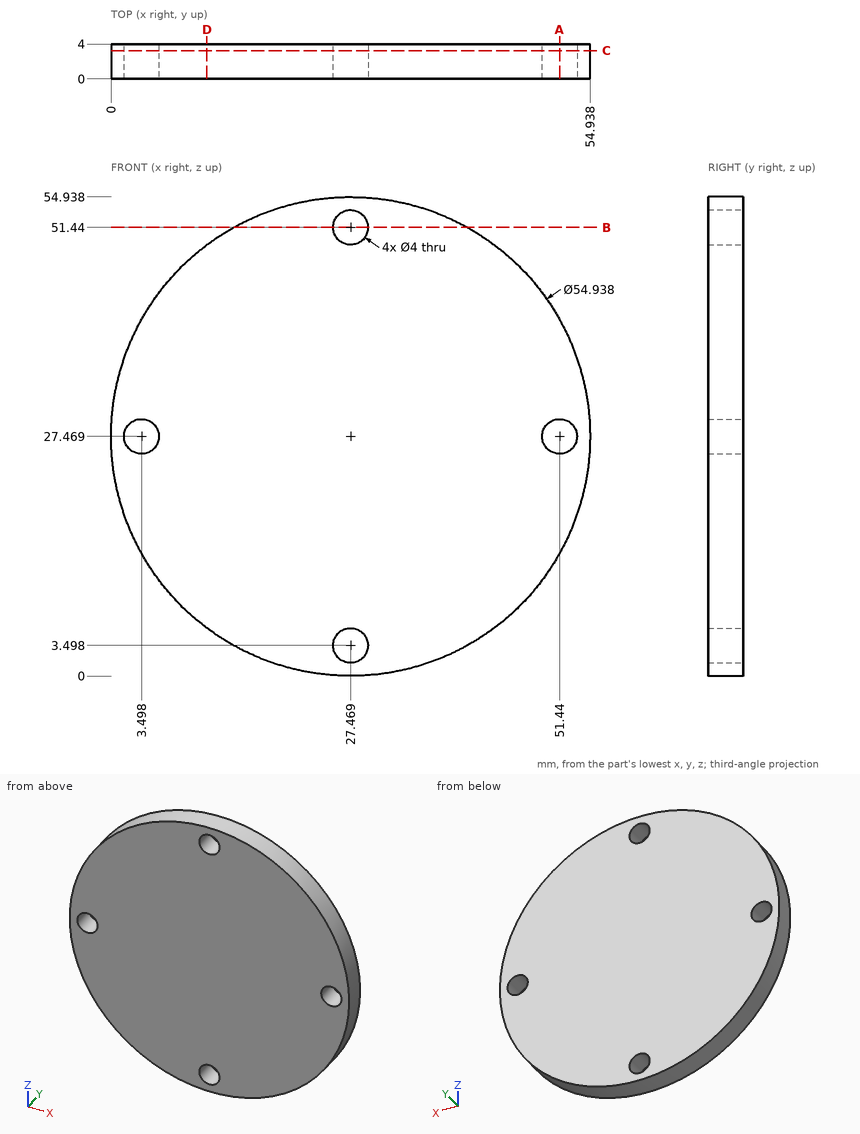
Can you work these out from the drawing? Everything is in mm from the part's minimum corner. Round coordinates to 2 decimals unless told otherwise and drop trailing zeros. Loops run counter-clockwise (first coordinate to the right, second up) from the corner with the lowest first, then second, coordinate; pieces in that order, holes last. Notation, with made-up numbers: (-3, 22) -> (8, 22) arc R23 ccw to (8, 32) -> close; hole circle Ø9 at (-10, 15.5). An arc over 180 degrees is marked (long way). Use CSV: the item, a comma, the result in double quotes.
(1) Suppose I cut it at A-A on x = 51.44. Write out the boundary of the cut face in (y, z).
Return value:
outline,"(0, 14.05) -> (4, 14.05) -> (4, 25.47) -> (0, 25.47) -> close; (0, 29.47) -> (4, 29.47) -> (4, 40.88) -> (0, 40.88) -> close"
(2) Will these pins go through, and if not, where does the flat tip stop? pin 1 Ø2.5 at (x, z) = (3.498, 27.469) entering from -Y; pin 2 Ø1.5 at (y, z) = (0.5, 13) entering from -X.
Return value:
pin 1,"passes through"
pin 2,"stops at x = 3.67"
(3) Suppose I cut it at D-D on x = 11. Write out the boundary of the cut face in (y, z).
Return value:
outline,"(0, 5.48) -> (4, 5.48) -> (4, 49.45) -> (0, 49.45) -> close"
(4) If I drill on probe 1 along Z at (x, y) = (3, 2.75); probe 2 along Z at (x, y) = (51, 0.85); probe 3 along X at (y, z) = (2.4, 4), over which ranges is the centre line in solid material (lowest first)? Write a range as [from, to].
Return value:
probe 1,"z = [14.99, 25.53], [29.41, 39.95]"
probe 2,"z = [13.3, 25.52], [29.42, 41.64]"
probe 3,"x = [13.19, 25.53], [29.4, 41.74]"
(5) Suppose I cut it at C-C on y = 3.25. Write out the boundary of the cut face in (x, z).
Return value:
outline,"circle Ø54.94 at (27.47, 27.47); hole circle Ø4 at (3.5, 27.47); hole circle Ø4 at (27.47, 3.5); hole circle Ø4 at (27.47, 51.44); hole circle Ø4 at (51.44, 27.47)"
(6) Suppose I cut it at B-B on z = 51.44. Write out the boundary of the cut face in (x, y), plus the area to 3 significant figures.
Return value:
outline,"(14.05, 0) -> (25.47, 0) -> (25.47, 4) -> (14.05, 4) -> close; (29.47, 0) -> (40.88, 0) -> (40.88, 4) -> (29.47, 4) -> close"
area,"91.3 mm²"
